from build123d import *

# Parameters (mm, degrees)
SKETCH1_W           = 381
SKETCH1_H           = 190.5
BOSS_EXTRUDE1_DEPTH = 6.35
SKETCH2_W           = 381
SKETCH2_H           = 31.75
BOSS_EXTRUDE2_DEPTH = 6.35
SKETCH3_R           = 3.175
CUT_EXTRUDE1_DEPTH  = 6.35
SKETCH4_R           = 3.175
CUT_EXTRUDE2_DEPTH  = 6.35
SKETCH5_R           = 3.175
CUT_EXTRUDE3_DEPTH  = 6.35


with BuildPart() as part:
    # Sketch1 → Boss-Extrude1 (new body)
    with BuildSketch(Plane(origin=(0, 0, 0), x_dir=(1, 0, 0), z_dir=(0, 1, 0))):
        Rectangle(SKETCH1_W, SKETCH1_H)
    extrude(amount=BOSS_EXTRUDE1_DEPTH)

    # Sketch2 → Boss-Extrude2 (add)
    with BuildSketch(Plane.XY.offset(95.25)):
        with Locations((0, 15.875)):
            Rectangle(SKETCH2_W, SKETCH2_H)
    extrude(amount=BOSS_EXTRUDE2_DEPTH)

    # Sketch3 → Cut-Extrude1 (cut)
    with BuildSketch(Plane.XY.offset(101.6)):
        with Locations((0, 19.05)):
            Circle(SKETCH3_R)
        with Locations((-127, 19.05)):
            Circle(SKETCH3_R)
        with Locations((127, 19.05)):
            Circle(SKETCH3_R)
    extrude(amount=-CUT_EXTRUDE1_DEPTH, mode=Mode.SUBTRACT)

    # Sketch4 → Cut-Extrude2 (cut)
    with BuildSketch(Plane.XZ):
        with Locations((0, 82.55)):
            Circle(SKETCH4_R)
        with Locations((-114.3, 82.55)):
            Circle(SKETCH4_R)
        with Locations((114.3, 82.55)):
            Circle(SKETCH4_R)
        with Locations((-114.3, -82.55)):
            Circle(SKETCH4_R)
        with Locations((114.3, -82.55)):
            Circle(SKETCH4_R)
    extrude(amount=-CUT_EXTRUDE2_DEPTH, mode=Mode.SUBTRACT)

    # Sketch5 → Cut-Extrude3 (cut)
    with BuildSketch(Plane.XZ):
        with Locations((174.8536, 57.15)):
            Circle(SKETCH5_R)
        with Locations((174.8536, 19.05)):
            Circle(SKETCH5_R)
        with Locations((174.8536, -19.05)):
            Circle(SKETCH5_R)
        with Locations((174.8536, -57.15)):
            Circle(SKETCH5_R)
        with Locations((-174.8536, -57.15)):
            Circle(SKETCH5_R)
        with Locations((-174.8536, -19.05)):
            Circle(SKETCH5_R)
        with Locations((-174.8536, 19.05)):
            Circle(SKETCH5_R)
        with Locations((-174.8536, 57.15)):
            Circle(SKETCH5_R)
    extrude(amount=-CUT_EXTRUDE3_DEPTH, mode=Mode.SUBTRACT)


solid = part.part
Work out the finished part from the listing and answer in its coordinate system (mm). A direction names the side the tool comes from. Give positions to 0.01 mm unless a question says otherwise; leave off trailing zeros. Write each loop counter-clockwise with the first axis right and the second up, starting at its lowest first coordinate (ties: lowest second). Pieces come first, ordered by that corner, then holes. Notation, with made-up numbers: (33.5, -14) - (63.5, -14) arc R16 cw to (63.5, 13) - close; hole circle Ø9 at (88.5, 57.5). An arc over 180 degrees is marked (long way). One line per item, written item: value. Start each with the question number.
1. Given pin 1 (4 mm diameter, centred on x = -76, y = 14, fed in from -Z), flat-ended and moving along its own axis, determine where the tip first touches the part or whether it passes through.
2. Find section B-B (z = -66). Write down the section's boundary in (x, y), then the cut area to 3 significant figures.
3. Find section A-A (x = -139). Write down the section's boundary in (y, z).
4. Find section C-C (y = 11). Write down the section's boundary in (x, z), then the cut area to 3 significant figures.
5. For faces 1 (the flat face through (190.5, 5, 17)), 2 (the flat face through (-3, 6.35, -1)), determine the directions among +Z, -Z, +X, -X, +Y, -Y from which every point of the face is accessible in a straight line to the end or side of a thin tool.
6. Consider probe 1 along Z at (x, y) = (-114, 5); probe 2 along Y at (x, z) = (0, 98) (3 decimals); probe 3 along X at (y, z) = (4, -19). Determine where each line is inside the solid, lowest interval first.
Geometry results:
1. pin 1: z = 95.25
2. outline: (-190.5, 0) - (190.5, 0) - (190.5, 6.35) - (-190.5, 6.35) - close
2. area: 2,420 mm2
3. outline: (0, -95.25) - (6.35, -95.25) - (6.35, 95.25) - (31.75, 95.25) - (31.75, 101.6) - (0, 101.6) - close
4. outline: (-190.5, 95.25) - (190.5, 95.25) - (190.5, 101.6) - (-190.5, 101.6) - close
4. area: 2,420 mm2
5. face 1: +Z, -Z, +X, +Y, -Y
5. face 2: -Z, +X, -X, +Y
6. probe 1: -95.25 to -85.71, -79.39 to 79.39, 85.71 to 101.6
6. probe 2: 0 to 15.875, 22.225 to 31.75
6. probe 3: -190.5 to -178.03, -171.68 to 171.68, 178.03 to 190.5
